Geometry: see drawing. Coordinates: mm, zero at the bounding-box minimum. A direction names the side the tool comes from. Coordinates: 2 decimals unless noted, no trailing zeros. Loops run counter-clockwise (first coordinate to the right, second up) from the corner with the lowest first, then second, coordinate; pieces in that order, holes last. Notation, with made-up numbers: (60.5, 1) -> (84.5, 1) arc R28 cw to (84.5, 25) -> close; hole circle Ø8 at (5, 73.5). An arc over 180 degrees is marked (long way). Answer as a JSON object with one key per item and string values.
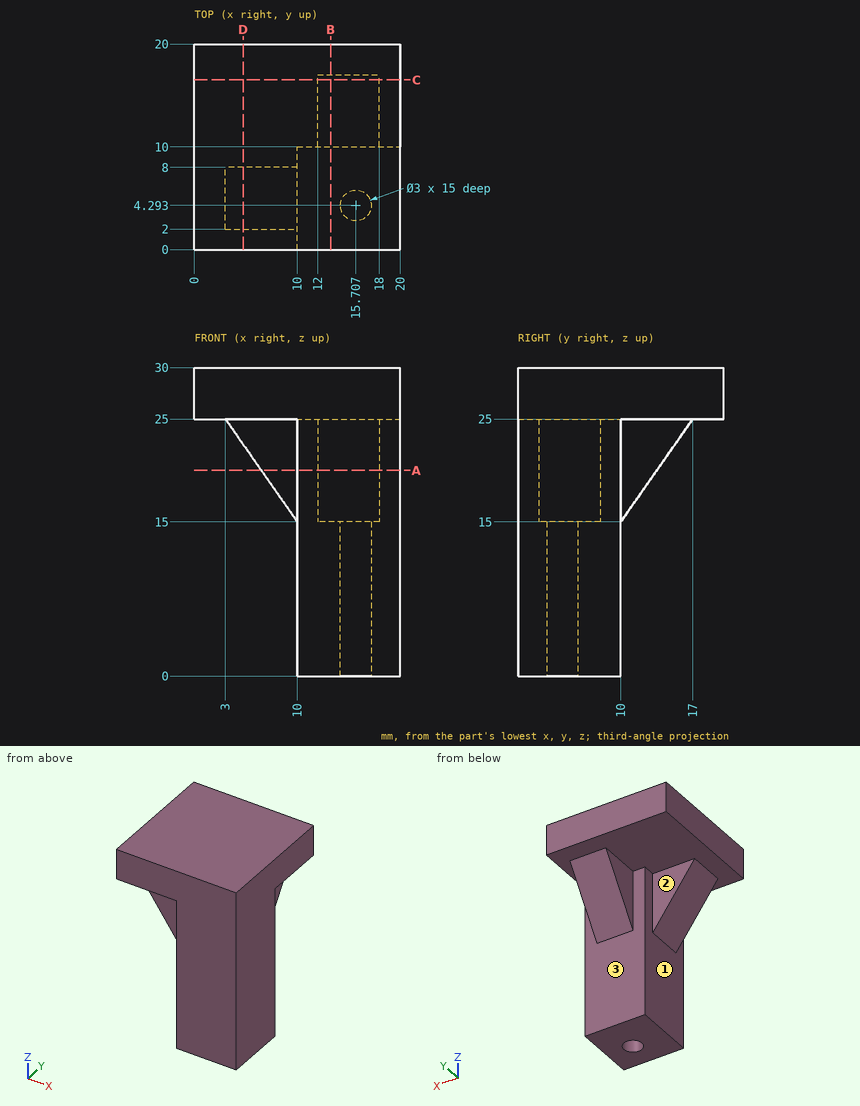
1. Line query: line 1 along Z through (x, y) = (8, 15.75); line 2 along X through (y, z) = (8.75, 11.25); line 3 along Y through (x, z) = (10.5, 2.25). Output: solid intervals per line, ascending.
Reply:
{"line 1": "z = 25 to 30", "line 2": "x = 10 to 20", "line 3": "y = 0 to 10"}
2. Section query D-D (x = 4.75). Return loops of the section in (y, z).
Reply:
{"outline": "(0, 25) -> (2, 25) -> (2, 22.5) -> (8, 22.5) -> (8, 25) -> (20, 25) -> (20, 30) -> (0, 30) -> close"}
3. Access query for the marked faces 1, 2 and 3. Directions: +Z, -Z, +X, -X, +Y, -Y. A direction counts if a zero-diameter tool reaches every point of the face in a straight line with its end or side. Return the directions, or none.
Reply:
{"face 1": "-Z, -X", "face 2": "-Z, -X, +Y", "face 3": "-Z, +Y"}
4. Section query B-B (x = 13.25). Return loops of the section in (y, z).
Reply:
{"outline": "(0, 0) -> (10, 0) -> (10, 15) -> (17, 25) -> (20, 25) -> (20, 30) -> (0, 30) -> close"}
5. Section query A-A (z = 20). Return loops of the section in (x, y), plus the area to 3 significant figures.
Reply:
{"outline": "(6.5, 2) -> (10, 2) -> (10, 0) -> (20, 0) -> (20, 10) -> (18, 10) -> (18, 13.5) -> (12, 13.5) -> (12, 10) -> (10, 10) -> (10, 8) -> (6.5, 8) -> close", "area": "142 mm2"}
6. Section query C-C (y = 16.5). Return loops of the section in (x, z).
Reply:
{"outline": "(0, 25) -> (12, 25) -> (12, 24.29) -> (18, 24.29) -> (18, 25) -> (20, 25) -> (20, 30) -> (0, 30) -> close"}
7. Pin query (flat end, axial travel): P1, Ø3.5, axis at y = 14, z = 18.5, coming from the +X side; P2, Ø5.5, axis at y = 15, z = 18, coming from the -X side; P3, Ø7.5, axis at x = 5.5, z = 19.5, coming from the +Y side. Return the tip coordinate at first contact, or that it passes through.
Reply:
{"P1": "stops at x = 18", "P2": "stops at x = 12", "P3": "stops at y = 8"}
